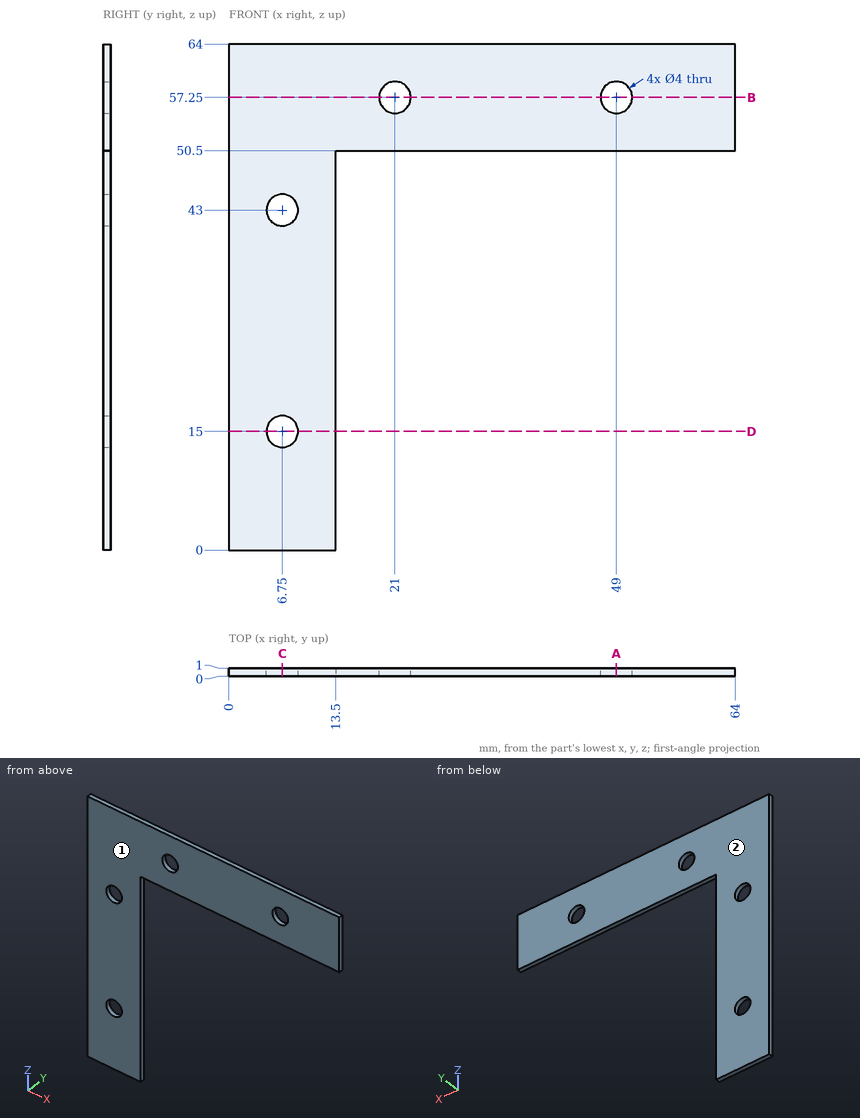
Drawing for the job (mm, zero at the part's lowest x, y, z). Give positions to 0.01 mm unless a question says otherwise; leave off trailing zeros. Order: outer loops, then holes, each group sorted by start corner. A loop starts at its lowest first (then second) coordinate and runs counter-clockwise, first axis right, second up. Notation, with made-up numbers: (-22, -28) - (21, -28) arc R14 cw to (21, -22) - close; hole circle Ø10 at (76.25, 45.25). An arc over 180 degrees is marked (long way). Write item = value, one per line. Start each with the question number.
1. Two-plate mould, pull along Y, no slides. Class the marked faces 1 and 2: pulls with the +Y half, pulls with the -Y half, needs draft (parallel to the pull), parting line crosses it, or undercut.
2. Probe line 1 along Z through (x, y) = (49, 0.4); line 2 along Z through (x, y) = (6.75, 0.45); line 3 along Z through (x, y) = (27, 0.7). List the from-to ranges inside material, lowest first.
3. Cut at C-C, the plane x = 6.75. List the corners of the cut face in (y, z), and give its area (3 significant figures).
4. Drop a flat-ended pin along its axis: P1, Ø0.5, axis at x = 41.5, y = 0.5, coming from the -Z side. Give the stop position or say it passes through.
5. Cut at B-B, the plane z = 57.25. List the corners of the cut face in (x, y), and give its area (3 significant figures).
6. Cut at A-A, the plane x = 49. List the corners of the cut face in (y, z).
7. Cut at D-D, the plane z = 15. List the corners of the cut face in (x, y), and give its area (3 significant figures).
Taken from the geometry:
q1.face_1 = pulls with the -Y half
q1.face_2 = pulls with the +Y half
q2.line_1 = 50.5 to 55.25, 59.25 to 64
q2.line_2 = 0 to 13, 17 to 41, 45 to 64
q2.line_3 = 50.5 to 64
q3.outline = (0, 0) - (1, 0) - (1, 13) - (0, 13) - close; (0, 17) - (1, 17) - (1, 41) - (0, 41) - close; (0, 45) - (1, 45) - (1, 64) - (0, 64) - close
q3.area = 56.0 mm²
q4.P1 = 50.5
q5.outline = (0, 0) - (19, 0) - (19, 1) - (0, 1) - close; (23, 0) - (47, 0) - (47, 1) - (23, 1) - close; (51, 0) - (64, 0) - (64, 1) - (51, 1) - close
q5.area = 56.0 mm²
q6.outline = (0, 50.5) - (1, 50.5) - (1, 55.25) - (0, 55.25) - close; (0, 59.25) - (1, 59.25) - (1, 64) - (0, 64) - close
q7.outline = (0, 0) - (4.75, 0) - (4.75, 1) - (0, 1) - close; (8.75, 0) - (13.5, 0) - (13.5, 1) - (8.75, 1) - close
q7.area = 9.50 mm²
